from build123d import *

# Parameters (mm, degrees)
SKETCH_R          = 2.5
SKETCH_R_2        = 2.499821
PAD_DEPTH         = 4
SKETCH001_R       = 5
SKETCH001_R_2     = 2.5
PAD001_DEPTH      = 7
FILLET_R          = 5
SKETCH002_W       = 12.9
SKETCH002_H       = 8.550953
POCKET_DEPTH      = 25.001
POCKET_DEPTH_BACK = 5.001
SKETCH003_R       = 5
SKETCH003_R_2     = 5.281206
POCKET001_DEPTH   = 1


with BuildPart() as part:
    # Sketch → Pad (new body)
    with BuildSketch(Plane.XY):
        with BuildLine():
            Line((-10, -5), (10, -5))
            ThreePointArc((10, -5), (15, -0.000187), (10.000374, 5))
            Line((7.5, 5), (10.000374, 5))
            Line((7.5, 25), (7.5, 5))
            Line((-7.5, 25), (7.5, 25))
            Line((-7.5, 25), (-7.5, 5))
            Line((-7.5, 5), (-9.999626, 5))
            ThreePointArc((-9.999626, 5), (-15, 0.000187), (-10, -5))
        make_face()
        with Locations((-10, 0)):
            Circle(SKETCH_R, mode=Mode.SUBTRACT)
        with Locations((10, 0)):
            Circle(SKETCH_R, mode=Mode.SUBTRACT)
        with Locations((0, 19)):
            Circle(SKETCH_R_2, mode=Mode.SUBTRACT)
        with Locations((0, 10)):
            Circle(SKETCH_R_2, mode=Mode.SUBTRACT)
    extrude(amount=PAD_DEPTH)

    # Sketch001 (on Face14 of Pad) → Pad001 (join)
    with BuildSketch(Plane.XY.offset(4)):
        with Locations((10, 0)):
            Circle(SKETCH001_R)
        with Locations((10, 0)):
            Circle(SKETCH001_R_2, mode=Mode.SUBTRACT)
        with Locations((-10, 0)):
            Circle(SKETCH001_R)
        with Locations((-10, 0)):
            Circle(SKETCH001_R_2, mode=Mode.SUBTRACT)
    extrude(amount=PAD001_DEPTH)

    # Fillet
    fillet_edges = [part.edges().sort_by_distance(p)[0] for p in [
        (-7.5, 25, 2),
        (7.5, 25, 2),
    ]]
    fillet(fillet_edges, radius=FILLET_R)

    # Sketch002 → Pocket (cut, two sides)
    with BuildSketch(Plane.XZ) as pocket_sk:
        with Locations((0, 8.275476)):
            Rectangle(SKETCH002_W, SKETCH002_H)
    extrude(amount=-POCKET_DEPTH, mode=Mode.SUBTRACT)
    extrude(pocket_sk.sketch, amount=POCKET_DEPTH_BACK, mode=Mode.SUBTRACT)

    # Sketch003 (on Face19 of Pocket) → Pocket001 (cut)
    with BuildSketch(Plane.XY.offset(4)):
        with Locations((0, 19)):
            Circle(SKETCH003_R)
        with Locations((0, 10)):
            Circle(SKETCH003_R_2)
    extrude(amount=-POCKET001_DEPTH, mode=Mode.SUBTRACT)


solid = part.part
Design review of the part built by this model. Coordinates are the model's own, in mm. A direction names the side the tool comes from. Coordinates: 2 decimals unless noted, no trailing zeros. Order: outer loops, then holes, each group sorted by start corner. A loop starts at its lowest first (then second) coordinate and runs counter-clockwise, first axis right, second up. Notation, with made-up numbers: (64, 80) - (110, 80) arc R22 ccw to (110, 91) - close; hole circle Ø5 at (19.25, 62.5). An arc over 180 degrees is marked (long way). Put each result on its own line as item: value.
1) Take a section at A-A, the plane z = 5. Give the boundary of the cut face in (x, y).
Response values:
outline: (-6.45, -3.52) - (-6.45, 3.52) arc R5 ccw (long way) to start; (6.45, -3.52) arc R5 ccw (long way) to (6.45, 3.52) - close; hole circle Ø5 at (-10, 0); hole circle Ø5 at (10, 0)
2) Insertion check: P1, Ø5.5, axis at y = 3.5, z = 9, coming from the -X side; P2, Ø6, axis at x = -2.5, y = -0.5, coming from the +Z side; P3, Ø4.5, axis at y = 14, z = 3, coming from the -X side. Each pin has a flat end and moves straight along its axis. Give the tip position at first contact, or say it passes through.
Response values:
P1: stops at x = -14.94
P2: stops at z = 4
P3: stops at x = -7.5
3) Wall thickness on L1, parallel to Y at x = 0, z = 1.7; L2, parallel to X at y = 10, z = 3.6; L3, parallel to X at y = 10, z = 2: over which ranges is each line inside the solid? List them lowest first. Write a range as from..to.
Response values:
L1: y = -5..7.5, 12.5..16.5, 21.5..25
L2: x = -7.5..-5.28, 5.28..7.5
L3: x = -7.5..-2.5, 2.5..7.5
4) Take a section at B-B, the plane y = 0. Give the boundary of the cut face in (x, z), and give its area (3 significant figures).
Response values:
outline: (-15, 0) - (-12.5, 0) - (-12.5, 11) - (-15, 11) - close; (-7.5, 0) - (7.5, 0) - (7.5, 11) - (6.45, 11) - (6.45, 4) - (-6.45, 4) - (-6.45, 11) - (-7.5, 11) - close; (12.5, 0) - (15, 0) - (15, 11) - (12.5, 11) - close
area: 130 mm²
5) The part is to be moulded in two halves that separate along Y. For faces 6 (the face through (0.183, 23.997, 3.507)), 7 (the face through (6, 23.57, 2.03)), 8 (the face through (-0.54, 7.56, 1.48)), 9 (the face through (13, 0, 11)), say which applies: released by +Y, released by -Y, zero draft, split by the parting line, or undercut.
Response values:
face 6: undercut
face 7: released by +Y
face 8: undercut
face 9: zero draft
6) Tool access review of faces 1 (the face through (7.5, 0.1, 5.4)), 2 (the face through (-9, 5, 2)), 3 (the face through (9, 5, 2)), 4 (the face through (-6.45, 0, 8)), 5 (the face through (-15, 0, 5)): name each direction out of +Z, -Z, +X, -X, +Y, -Y from which nothing blocks a thin tool from reaching the whole face with its end or side.
Response values:
face 1: +Z, -Z
face 2: +Z, -Z, -X, +Y
face 3: +Z, -Z, +X, +Y
face 4: +Z, +Y, -Y
face 5: +Z
7) Take a section at D-D, the plane x = 8.5. Give the boundary of the cut face in (y, z).
Response values:
outline: (-5, 0) - (-2, 0) - (-2, 11) - (-4.77, 11) - (-4.77, 4) - (-5, 4) - close; (2, 0) - (5, 0) - (5, 4) - (4.77, 4) - (4.77, 11) - (2, 11) - close
8) Take a section at C-C, the plane y = 10. Give the boundary of the cut face in (x, z), and give its area (3 significant figures).
Response values:
outline: (-7.5, 0) - (-2.5, 0) - (-2.5, 3) - (-5.28, 3) - (-5.28, 4) - (-7.5, 4) - close; (2.5, 0) - (7.5, 0) - (7.5, 4) - (5.28, 4) - (5.28, 3) - (2.5, 3) - close
area: 34.4 mm²
